```python
from build123d import *

# Parameters (mm, degrees)
F0_W     = 74.744492
F0_H     = 116.611682
F0_R     = 19.451918
F1_DEPTH = 25.4
F2_DEPTH = 23.622
F4_DEPTH = 74.745493


with BuildPart() as f1:
    # F0 (on Top) → F1 (new body)
    with BuildSketch(Plane.XY):
        Rectangle(F0_W, F0_H)
        Circle(F0_R, mode=Mode.SUBTRACT)
        Circle(F0_R)
    extrude(amount=F1_DEPTH)

    # F0 (on Top) → F2 (join)
    with BuildSketch(Plane.XY):
        Circle(F0_R)
    extrude(amount=-F2_DEPTH)

    # F3 (on face) → F4 (cut, through all)
    with BuildSketch(Plane.YZ.offset(37.372246)):
        Polygon((-19.451918, 0), (-19.451918, -23.622), (19.451918, -23.622), align=None)
    extrude(amount=-F4_DEPTH, mode=Mode.SUBTRACT)


solid = f1.part
```
Verification items for the finished model (mm, model axes). Coordinates: 2 decimals unless noted, no trailing zeros. Loops run counter-clockwise (first coordinate to the right, second up) from the corner with the lowest first, then second, coordinate; pieces in that order, holes last. Notation, with made-up numbers: (14.5, 35) -> (54.5, 35) arc R17 ccw to (54.5, 52) -> close; hole circle Ø1 at (-30, 80). An arc over 180 degrees is marked (long way). Put each result on its own line as item: value.
1. Thickness scan on line 1 (Z direction, x = 2.5, y = -50.5); line 2 (Y direction, x = 18, z = -6); line 3 (Y direction, x = -3, z = -2). Record the ranges inside material, lowest first.
Result set:
line 1: z = 0 to 25.4
line 2: y = -7.37 to 7.37
line 3: y = -16.16 to 19.22
2. Section check D-D, the plane y = -27. Record the boundary of the cut face in (x, z).
Result set:
outline: (-37.37, 0) -> (37.37, 0) -> (37.37, 25.4) -> (-37.37, 25.4) -> close
3. Section check B-B, the plane x = 17. Record the boundary of the cut face in (y, z), then the cut area to 3 significant figures.
Result set:
outline: (-58.31, 0) -> (-9.45, 0) -> (-9.45, -6.07) -> (9.45, -17.55) -> (9.45, 0) -> (58.31, 0) -> (58.31, 25.4) -> (-58.31, 25.4) -> close
area: 3,190 mm^2
4. Section check C-C, the plane z = -19. Record the boundary of the cut face in (x, y).
Result set:
outline: (-15.43, 11.84) -> (15.43, 11.84) arc R19.45 ccw to start
5. Gauge pin test, flat end, axial feed: P1, Ø2, axis at x = -12, z = -4.5, coming from the +Y side. Record the tip position at first contact, or that the pin passes through.
Result set:
P1: stops at y = 16.04
6. Section check A-A, the plane y = 0. Record the boundary of the cut face in (x, z), then the cut area to 3 significant figures.
Result set:
outline: (-37.37, 0) -> (-19.45, 0) -> (-19.45, -11.81) -> (19.45, -11.81) -> (19.45, 0) -> (37.37, 0) -> (37.37, 25.4) -> (-37.37, 25.4) -> close
area: 2,360 mm^2
7. Mould release check, pull along Z, two halves, no side actions. Record for faces 1 (the face through (0.272, 0.272, -11.976)), 2 (the face through (-1, 1, 25.4)), 3 (the face through (-1, -58.306, 13)): pulls with the +Z half, pulls with the -Z half, needs draft (parallel to the pull), parting line crosses it, or undercut.
Result set:
face 1: pulls with the -Z half
face 2: pulls with the +Z half
face 3: needs draft
